from build123d import *

# Parameters (mm, degrees)
PAD_DEPTH           = 14
POCKET_DEPTH        = 24.001
POCKET_DEPTH_BACK   = -24.001
SKETCH002_W         = 1.5
SKETCH002_H         = 1
POCKET001_DEPTH     = 10.001
LINEARPATTERN_COUNT = 15
LINEARPATTERN_PITCH = 2
POCKET002_DEPTH     = 8.001
POCKET003_DEPTH     = 6


with BuildPart() as part:
    # Sketch → Pad (new body)
    with BuildSketch(Plane.XY):
        Polygon((12.5, 24), (12.5, -24), (5.15, -24), (4.5, -23.35), (4.5, -15), (-9.1, -15), (-11, -13.1), (-11, 13.1), (-9.1, 15), (4.5, 15), (4.5, 23.35), (5.15, 24), align=None)
    extrude(amount=PAD_DEPTH)

    # Sketch001 → Pocket (cut, two sides)
    with BuildSketch(Plane.XZ) as pocket_sk:
        Polygon((6.5, 15), (6.5, 14.23), (4.5, 12.23), (4.5, 12), (1.64, 12), (0.165531, 10.525531), (-0.05, 8.062), (-0.05, 4), (-0.8, 4), (-0.8, 8.64), (-1.022434, 11.182434), (-1.84, 12), (-3.36, 12), (-4.834469, 10.525531), (-5.05, 8.062), (-5.05, 4), (-5.8, 4), (-5.8, 8.64), (-6.022434, 11.182434), (-6.84, 12), (-12, 12), (-12, 15), align=None)
    extrude(amount=-POCKET_DEPTH, mode=Mode.SUBTRACT)
    extrude(pocket_sk.sketch, amount=-POCKET_DEPTH_BACK, mode=Mode.SUBTRACT)

    # Sketch002 → Pocket001 (cut, through all)
    with BuildSketch(Plane.XY.offset(4)):
        with Locations((-6.1, 14.5)):
            Rectangle(SKETCH002_W, SKETCH002_H)
        with Locations((-1.05, 13.5)):
            Rectangle(SKETCH002_W, SKETCH002_H)
    pocket001 = extrude(amount=POCKET001_DEPTH, mode=Mode.SUBTRACT)

    # LinearPattern: Pocket001 ×15
    with Locations(*[(0, -i * LINEARPATTERN_PITCH, 0) for i in range(1, LINEARPATTERN_COUNT)]):
        add(pocket001, mode=Mode.SUBTRACT)

    # Sketch003 → Pocket002 (cut, through all)
    with BuildSketch(Plane.YZ.offset(4.5)):
        with BuildLine():
            ThreePointArc((-19.5, 8.65), (-21.15, 7), (-19.5, 5.35))
            Line((-19.5, 5.35), (-19, 5.35))
            ThreePointArc((-19, 5.35), (-17.35, 7), (-19, 8.65))
            Line((-19, 8.65), (-19.5, 8.65))
        make_face()
        with BuildLine():
            ThreePointArc((19, 8.65), (17.35, 7), (19, 5.35))
            Line((19, 5.35), (19.5, 5.35))
            ThreePointArc((19.5, 5.35), (21.15, 7), (19.5, 8.65))
            Line((19.5, 8.65), (19, 8.65))
        make_face()
    extrude(amount=POCKET002_DEPTH, mode=Mode.SUBTRACT)

    # Sketch004 → Pocket003 (cut)
    with BuildSketch(Plane.YZ.offset(4.5)):
        with BuildLine():
            ThreePointArc((-19.5, 10.1), (-22.6, 7), (-19.5, 3.9))
            Line((-19.5, 3.9), (-19, 3.9))
            ThreePointArc((-19, 3.9), (-15.9, 7), (-19, 10.1))
            Line((-19, 10.1), (-19.5, 10.1))
        make_face()
        with BuildLine():
            ThreePointArc((19, 10.1), (15.9, 7), (19, 3.9))
            Line((19, 3.9), (19.5, 3.9))
            ThreePointArc((19.5, 3.9), (22.6, 7), (19.5, 10.1))
            Line((19.5, 10.1), (19, 10.1))
        make_face()
    extrude(amount=POCKET003_DEPTH, mode=Mode.SUBTRACT)


solid = part.part
Work out the finished part from the listing and answer in its coordinate system (mm). A direction names the side the tool comes from. Round coordinates to 2 decimals unless told otherwise and drop trailing zeros. Loops run counter-clockwise (first coordinate to the right, second up) from the corner with the lowest first, then second, coordinate; pieces in that order, holes last. Notation, with made-up numbers: M 17.5,-38 L 63.5,-38 A35 cw 63.5,1 Z; hole C 60,5 d7. An arc over 180 degrees is marked long. One line per question, with ' | ' between items. Start each with the question number.
(1) Find the intervals of material crossed by line 1 (X direction, y = -8.5, z = 4.25); line 2 (Y direction, x = 7, z = 6.75); line 3 (X direction, y = -12.5, z = 11.25), in increasing order.
(2) A cutting plane is placed at B-B on y = 6.5. Write down the section's boundary in (x, z), plus the area to 3 significant figures.
(3) A cutting plane is placed at A-A on y = -20. Write down the section's boundary in (x, z).
(4) A cutting plane is placed at C-C on z = 1. Write down the section's boundary in (x, y), plus the area to 3 significant figures.
(5) A cutting plane is placed at D-D on z = 6. Give the number of separate pieces and of enclosed holes in the cut face, plus the area to 3 significant figures.
(6) Flat-ended cylindrical pins translate along their axes: pin 1 Ø1.1 at (x, z) = (-1.5, 8.5) entering from +Y; pin 2 Ø0.5 at (x, z) = (-1.5, 9) entering from -Y; pin 3 Ø1 at (x, y) = (-5, 0) entering from +Z. Find the tip coordinate at first contact, or state that the pin passes through.
(7) For a pull along X with two mould halves and no side action, classify faces 5 (the face through (-0.91, -1.49, 9.89)), 6 (the face through (-6.85, 8.5, 7.9)), 7 (the face through (7.5, 22.6, 6.9)) as released by +X, released by -X, zero draft, split by the parting line, or undercut.
(8) A tool of negligible diameter and unlimited length cuts with its end or side. For faces 1 (the face through (11.49, -17.35, 6.96)), 2 (the face through (-0.05, 0, 6)), 3 (the face through (-6, -11, 8)), 4 (the face through (3, 0, 12)), from which of +Z, -Z, +X, -X, +Y, -Y can it reach the whole face along a straight path? Write none if from no direction.
Geometry check:
1) line 1: x = -11 to -5.8, -5.05 to -1.8, -0.05 to 12.5 | line 2: y = -24 to -22.59, -15.91 to 15.91, 22.59 to 24 | line 3: x = -11 to -6.09, -4.11 to -1.8, 0.89 to 12.5
2) outline: M -11,0 L 12.5,0 L 12.5,14 L 6.27,14 L 4.5,12.23 L 4.5,12 L 1.64,12 L 0.17,10.53 L -0.05,8.06 L -0.05,4 L -0.8,4 L -0.8,8.64 L -1.02,11.18 L -1.84,12 L -3.36,12 L -4.83,10.53 L -5.05,8.06 L -5.05,4 L -6.85,4 L -6.85,12 L -11,12 Z | area: 272 mm²
3) outline: M 4.5,0 L 12.5,0 L 12.5,5.43 L 10.5,5.43 L 10.5,3.94 L 4.5,3.94 Z; M 4.5,10.06 L 10.5,10.06 L 10.5,8.57 L 12.5,8.57 L 12.5,14 L 6.27,14 L 4.5,12.23 Z
4) outline: M -11,-13.1 L -9.1,-15 L 4.5,-15 L 4.5,-23.35 L 5.15,-24 L 12.5,-24 L 12.5,24 L 5.15,24 L 4.5,23.35 L 4.5,15 L -9.1,15 L -11,13.1 Z | area: 845 mm²
5) separate pieces: 5 | enclosed holes: 0 | area: 680 mm²
6) pin 1: stops at y = 15 | pin 2: stops at y = -14 | pin 3: stops at z = 10.86
7) face 5: undercut | face 6: undercut | face 7: zero draft
8) face 1: +X, -X | face 2: +Z, +Y, -Y | face 3: +Z | face 4: +Z, -X, +Y, -Y
